Geometry: final body of the model. Coordinates: model frame, mm. A direction names the side the tool comes from. Give positions to 0.01 mm unless a question says otherwise; leave off trailing zeros. Loops run counter-clockwise (first coordinate to the right, second up) from the corner with the lowest first, then second, coordinate; pieces in that order, holes last.
Solid Edge part; units mm, degrees
sketch "Sketch1" plane through (0, 0, 0) normal (0, -1, 0) x (1, 0, 0)
  circle A0 centre (0, 0) radius 30
extrude "Protrusion1" add sketch "Sketch1" against normal blind 10
sketch "Sketch2" plane through (0, 10, 0) normal (0, 1, 0) x (0, 0, 1)
  circle A0 centre (-26.5, 0) radius 1.6
extrude "Cutout1" cut sketch "Sketch2" against normal up to next
pattern_circular "Pattern1" count 6 over 360 about axis through (0, 10, 0) along (0, -1, 0) of "Cutout1"
sketch "Sketch3" plane through (0, 10, 0) normal (0, 1, 0) x (0, 0, 1)
  line L0 (-27.1295, -30) -> (30.6259, -30)
  line L1 (30.6259, -30) -> (30.6259, -27)
  line L2 (30.6259, -27) -> (-27.1295, -27)
  line L3 (-27.1295, -27) -> (-27.1295, -30)
  line L4 (-24.9621, 30) -> (24.2465, 30)
  line L5 (24.2465, 30) -> (24.2465, 27)
  line L6 (24.2465, 27) -> (-24.9621, 27)
  line L7 (-24.9621, 27) -> (-24.9621, 30)
  dimension "D1" = 30.6259
extrude "Cutout2" cut sketch "Sketch3" against normal up to next
sketch "Sketch4" plane through (0, 0, 0) normal (0, -1, 0) x (0, 0, -1)
  circle A0 centre (0, 0) radius 6.45
extrude "ExtrudedCutout_3" cut sketch "Sketch4" against normal blind 5
chamfer "Chamfer_1" distance 1.5 angle 45 1 edges at (0, 0, 6.45)
Item 1: Section query B-B on z = 0. Return loops of the section in (x, y), plus the area to 3 significant figures.
Values follow:
outline: (-27, 0) - (-7.95, 0) - (-6.45, 1.5) - (-6.45, 5) - (6.45, 5) - (6.45, 1.5) - (7.95, 0) - (27, 0) - (27, 10) - (-27, 10) - close
area: 473 mm2
Item 2: Section query A-A on x = 0. Return loops of the section in (y, z).
Values follow:
outline: (0, -30) - (10, -30) - (10, -28.1) - (0, -28.1) - close; (0, -24.9) - (10, -24.9) - (10, 24.9) - (0, 24.9) - (0, 7.95) - (1.5, 6.45) - (5, 6.45) - (5, -6.45) - (1.5, -6.45) - (0, -7.95) - close; (0, 28.1) - (10, 28.1) - (10, 30) - (0, 30) - close
Item 3: Pin query (flat end, axial travel): pin 1 (2 mm diameter, centred on y = 4, z = -19, fed in from +X); pin 2 (2.5 mm diameter, centred on x = 0, z = 26.5, fed in from +Y); pin 3 (14 mm diameter, centred on x = 0.5, z = 0.5, fed in from -Y); pin 4 (12 mm diameter, centred on x = 21, z = 10, fed in from -Y). Return the tip coordinate at first contact, or that it passes through.
Values follow:
pin 1: stops at x = 24
pin 2: passes through
pin 3: stops at y = 0.24
pin 4: stops at y = 0
Item 4: Section query C-C on y = 7.5. Return loops of the section in (x, z), plus the area to 3 significant figures.
Values follow:
outline: (-27, -13.08) arc R30 ccw to (27, -13.08) - (27, 13.08) arc R30 ccw to (-27, 13.08) - close; hole circle Ø3.2 at (-22.95, -13.25); hole circle Ø3.2 at (-22.95, 13.25); hole circle Ø3.2 at (0, -26.5); hole circle Ø3.2 at (0, 26.5); hole circle Ø3.2 at (22.95, -13.25); hole circle Ø3.2 at (22.95, 13.25)
area: 2,670 mm2
Item 5: Draft query along X for faces 3 (the face through (-6.297, 3.226, 1.398)), 4 (the face through (-27, 5, 0)), 5 (the face through (0, 5, 30)). Return one class per face: +X half, -X half, draft (parallel to the pull), parting line (faces both ways), or undercut.
Values follow:
face 3: undercut
face 4: -X half
face 5: parting line
Item 6: Ray query, probe 1 along X at (y, z) = (6, -13.25); probe 2 along Z at (x, y) = (23, 3); probe 3 along X at (y, z) = (6, -12.5). Return the intervals inside material, ascending.
Values follow:
probe 1: x = -26.92 to -24.55, -21.35 to 21.35, 24.55 to 26.92
probe 2: z = -19.26 to -14.85, -11.65 to 11.65, 14.85 to 19.26
probe 3: x = -27 to -24.36, -21.54 to 21.54, 24.36 to 27
Item 7: Set-up query: faces 1 (the face through (24.536, 5.07, 13.042)), 2 (the face through (0, 5, 0)). Return all of +Z, -Z, +X, -X, +Y, -Y with unobstructed straight access to the full face (end or side cutting, diameter ignored); none if empty.
Values follow:
face 1: +Y, -Y
face 2: -Y
Item 8: Section query D-D on z = -26.5. Return loops of the section in (x, y), plus the area to 3 significant figures.
Values follow:
outline: (-14.06, 0) - (-1.6, 0) - (-1.6, 10) - (-14.06, 10) - close; (1.6, 0) - (14.06, 0) - (14.06, 10) - (1.6, 10) - close
area: 249 mm2
